Drawing for the job (mm, zero at the part's lowest x, y, z). Give positions to 0.01 mm unless a question says otherwise; leave off trailing zeros. Write each loop counter-clockwise with the first axis right and the second up, starting at its lowest first coordinate (ties: lowest second). Pieces come first, ordered by that corner, then holes. Notation, with made-up numbers: M 7,16 L 21,16 A28 cw 21,47 Z; hole C 83.25,-1.5 d11. An arc over 180 degrees is marked long. Write item = value, one per line. Start each with the question number.
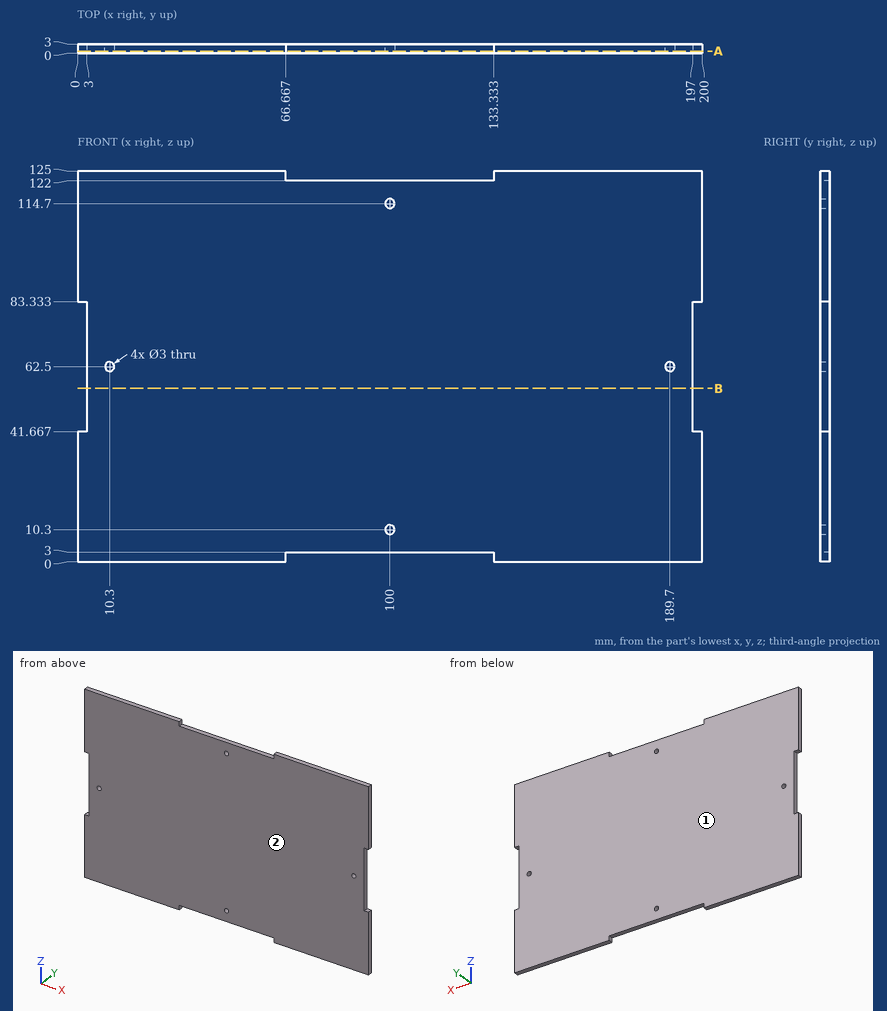
Q1. Two-plate mould, pull along Y, no slides. Class the marked faces 1 and 2: +Y half, -Y half, draft (parallel to the pull), parting line (faces both ways), or undercut.
Q2. Slice it at B-B (z = 55.5). Give the cut face in (x, y).
Q3. Drop flat-ended pins along their axis: P1, Ø0.9, axis at x = 112, y = 1, coming from the +Z side; P2, Ø1.8, axis at x = 100, z = 10.3, coming from the +Y side; P3, Ø0.9, axis at y = 1.5, z = 71, coming from the +X side; P4, Ø0.9, axis at y = 1, z = 56, coming from the -X side. Give the stop position or say it passes through.
Q4. Slice it at A-A (y = 0.7). Give the cut face in (x, z).
Q5. Probe line 1 along Z through (x, y) = (100, 2.35); line 2 along Z through (x, y) = (10.3, 1.55); line 3 along Z through (x, y) = (71.5, 1.55). List the from-to ranges inside material, lowest first.
Working result:
q1.face_1 = +Y half
q1.face_2 = -Y half
q2.outline = M 3,0 L 197,0 L 197,3 L 3,3 Z
q3.P1 = 122
q3.P2 = through
q3.P3 = 197
q3.P4 = 3
q4.outline = M 0,0 L 66.67,0 L 66.67,3 L 133.33,3 L 133.33,0 L 200,0 L 200,41.67 L 197,41.67 L 197,83.33 L 200,83.33 L 200,125 L 133.33,125 L 133.33,122 L 66.67,122 L 66.67,125 L 0,125 L 0,83.33 L 3,83.33 L 3,41.67 L 0,41.67 Z; hole C 10.3,62.5 d3; hole C 100,10.3 d3; hole C 100,114.7 d3; hole C 189.7,62.5 d3
q5.line_1 = 3 to 8.8, 11.8 to 113.2, 116.2 to 122
q5.line_2 = 0 to 61, 64 to 125
q5.line_3 = 3 to 122
